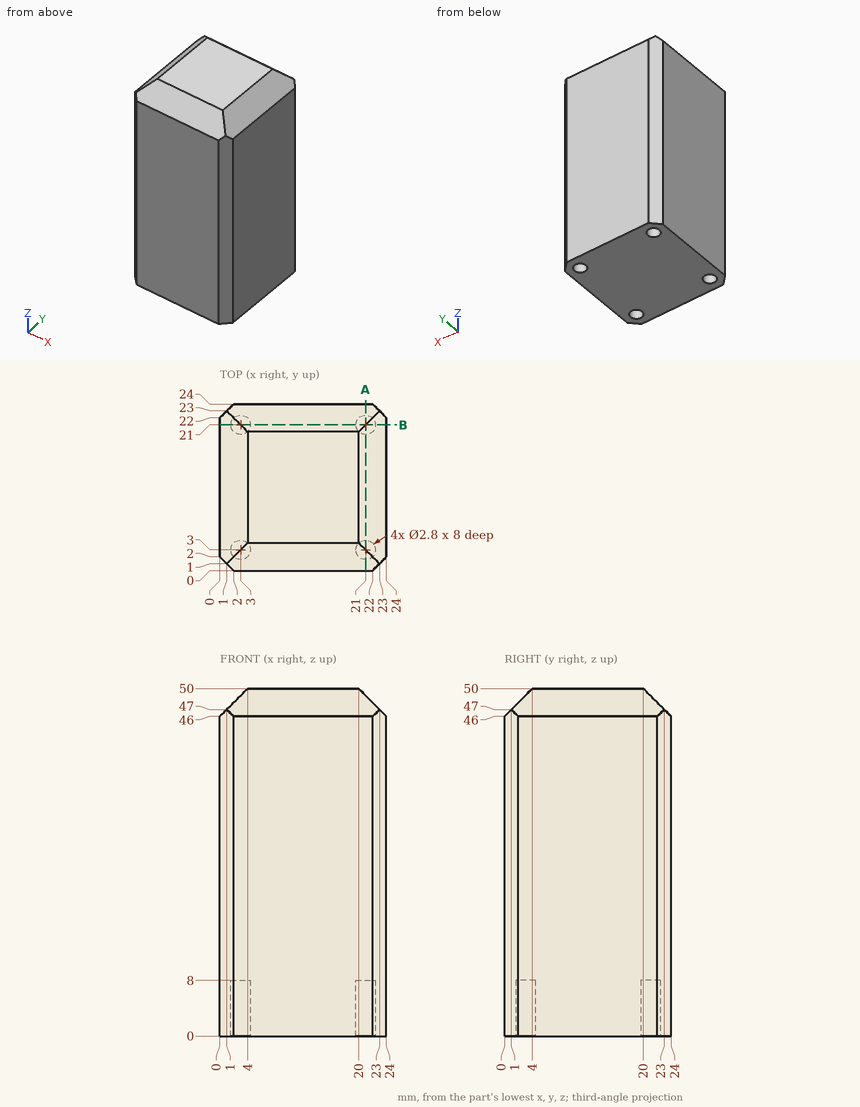
Verification items for this drawing (mm, ordinates from the low corner). Round coordinates to 2 decimals unless told otherwise and drop trailing zeros. Loops run counter-clockwise (first coordinate to the right, second up) from the corner with the lowest first, then second, coordinate; pieces in that order, holes last. Notation, with made-up numbers: (63.5, 22) - (77.5, 22) arc R12 ccw to (77.5, 34) - close; hole circle Ø2 at (62, 37). An arc over 180 degrees is marked (long way). Answer as CSV lines item,"result". Start each with the question number.
Item 1: Section check A-A (x = 21). Record the boundary of the cut face in (y, z), and give its area (3 significant figures).
Item 2: Scan lines: line 1 (Y direction, x = 21, z = 6); line 2 (Y direction, x = 20.5, z = 4); line 3 (Z direction, x = 4, y = 1.5). Record each from-to range of solid material in increasing order. Write a range as [from, to].
Item 3: Depth check by flat-ended pin: P1, Ø2, axis at x = 21, y = 3, coming from the -Z side. Enter the tip coordinate at first touch or a pass-through.
Report:
1,outline,"(0, 0) - (1.6, 0) - (1.6, 8) - (4.4, 8) - (4.4, 0) - (19.6, 0) - (19.6, 8) - (22.4, 8) - (22.4, 0) - (24, 0) - (24, 46) - (21, 49) - (3, 49) - (0, 46) - close"
1,area,"1,120 mm2"
2,line 1,"y = [0, 1.6], [4.4, 19.6], [22.4, 24]"
2,line 2,"y = [0, 1.69], [4.31, 19.69], [22.31, 24]"
2,line 3,"z = [0, 47.5]"
3,P1,"stops at z = 8"
